Autodesk Inventor part; units mm, degrees
ref_plane "YZ Plane" through (0, 0, 0) normal (1, 0, 0) x (0, 1, 0)
ref_plane "XZ Plane" through (0, 0, 0) normal (0, 1, 0) x (-1, 0, 0)
ref_plane "XY Plane" through (0, 0, 0) normal (0, 0, 1) x (1, 0, 0)
sketch "Sketch1" plane through (0, 0, 0) normal (0, 0, 1) x (1, 0, 0)
  circle A0 centre (0, 0) radius 12.5
  dimension "d0" = 25
extrude "Extrusion1" add sketch "Sketch1" along normal blind 20
sketch "Sketch2" plane through (0, 0, 0) normal (0, 0, -1) x (-1, 0, 0)
  circle A0 centre (0, 0) radius 4.5
  circle A1 centre (0, 0) radius 7.5
  dimension "d3" = 9
  dimension "d4" = 3
extrude "Extrusion2" add sketch "Sketch2" along normal blind 98
sketch "Sketch3" plane through (0, 0, 20) normal (0, 0, 1) x (1, 0, 0)
  circle A0 centre (0, 0) radius 4.5
  dimension "d7" = 9
extrude "Extrusion3" cut sketch "Sketch3" against normal through all
sketch "Sketch4" plane through (0, 0, 20) normal (0, 0, 1) x (1, 0, 0)
  circle A0 centre (0, 0) radius 9.5
  dimension "d10" = 19
extrude "Extrusion4" cut sketch "Sketch4" against normal blind 15.44
properties part number "Adapter" material "Stainless Steel"
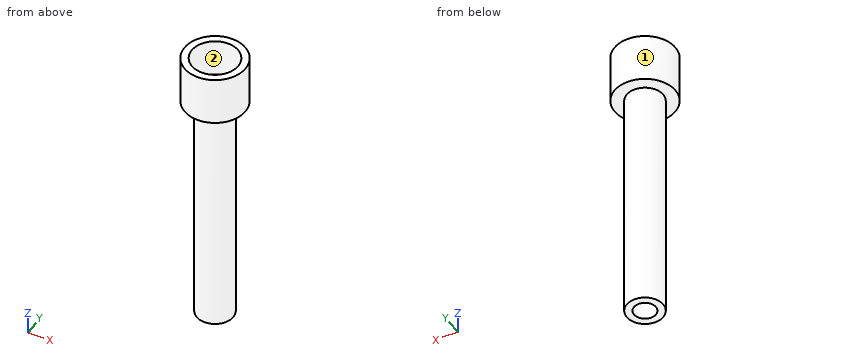
Model file for the job. Use its own axes, mm. Face numbers are marked on the shaded views. Round coordinates to 2 decimals unless told otherwise and drop trailing zeros. Order: outer loops, then holes, each group sorted by start corner. A loop starts at its lowest first (then second) coordinate and runs counter-clockwise, first axis right, second up.
(1) Pin check, flat tips, straight feed: pin 1 (12 mm diameter, centred on y = 3.5, z = 5, fed in from +X); pin 2 (5 mm diameter, centred on x = 5.5, z = -27.5, fed in from -Y); pin 3 (4 mm diameter, centred on y = -0.5, z = -55, fed in from +X); pin 4 (6 mm diameter, centred on x = -10, z = 0, fed in from +Y). Stop position of each tip, or through.
(2) Drill centre lines: line 1 (Y direction, x = 0, z = 9.75); line 2 (Y direction, x = 0, z = -54); line 3 (X direction, y = 0.25, z = -59). Where is each one in solid material? Low to high.
(3) Band-saw the part on D-D (x = 8.5). List the corners of the cut face in (y, z).
(4) Pull direction X, two halves, no side cores. Call the marked faces 1 and 2: released by +X, released by -X, zero draft, split by the parting line, or undercut.
(5) Band-saw the part on C-C (z = -81.5). List the corners of the cut face in (x, y).
(6) Band-saw the part on A-A (y = 0). List the corners of the cut face in (x, z), then the cut area to 3 significant figures.
Verdict:
1. pin 1: stops at x = 12.5
1. pin 2: stops at y = -6.87
1. pin 3: stops at x = 7.5
1. pin 4: stops at y = 10.36
2. line 1: y = -12.5 to -9.5, 9.5 to 12.5
2. line 2: y = -7.5 to -4.5, 4.5 to 7.5
2. line 3: x = -7.5 to -4.49, 4.49 to 7.5
3. outline: (-9.17, 0) - (9.17, 0) - (9.17, 20) - (4.24, 20) - (4.24, 4.56) - (-4.24, 4.56) - (-4.24, 20) - (-9.17, 20) - close
4. face 1: split by the parting line
4. face 2: undercut
5. outline: circle Ø15 at (0, 0); hole circle Ø9 at (0, 0)
6. outline: (-12.5, 0) - (-7.5, 0) - (-7.5, -98) - (-4.5, -98) - (-4.5, 4.56) - (-9.5, 4.56) - (-9.5, 20) - (-12.5, 20) - close; (4.5, -98) - (7.5, -98) - (7.5, 0) - (12.5, 0) - (12.5, 20) - (9.5, 20) - (9.5, 4.56) - (4.5, 4.56) - close
6. area: 754 mm2
